For this review, take the finished solid that the model builds, in its own axes (mm). A direction names the side the tool comes from. Round coordinates to 2 decimals unless told otherwise and drop trailing zeros. Order: outer loops, then holes, each group sorted by start corner. A loop starts at its lowest first (then second) coordinate and runs counter-clockwise, first axis right, second up. Notation, with made-up numbers: M 47.25,27 L 75.25,27 A14 cw 75.25,43 Z; hole C 34,71 d3. An arc over 180 degrees is marked long. Put each result on its own line as item: value.
from build123d import *

# Parameters (mm, degrees)
ESQUISSE2_R               = 3.5
ESQUISSE2_R_2             = 1.25
ESQUISSE2_R_3             = 1.5
ESQUISSE2_W               = 8
ESQUISSE2_H               = 3
ESQUISSE2_W_2             = 5.5
T_LE_DE_BASE_PLI_E1_DEPTH = 3


# Sheet-metal steps are written as plain solids
with BuildPart() as part:
    # Esquisse2 → Tôle de base pliée1 (new body)
    with BuildSketch(Plane.XY):
        with BuildLine():
            Line((-80.674813436, 13.65), (-5.9, 13.65))
            ThreePointArc((-5.9, 13.65), (0, 7.75), (-5.9, 1.85))
            Line((-5.9, 1.85), (-80.674813436, 1.85))
            ThreePointArc((-80.674813436, 1.85), (-85.688411127, 8.665e-06), (-90.707519116, 1.834997692))
            ThreePointArc((-90.707519116, 1.834997692), (-94.311259808, 3.720569786), (-98.375041782, 3.887917208))
            ThreePointArc((-98.375041782, 3.887917208), (-102.999999988, 7.750307003), (-98.374437627, 11.611973247))
            ThreePointArc((-98.374437627, 11.611973247), (-94.311297529, 11.778940178), (-90.708236779, 13.664394674))
            ThreePointArc((-90.708236779, 13.664394674), (-85.688881301, 15.499992024), (-80.674813436, 13.65))
        make_face()
        with Locations((-85.7, 7.75)):
            Circle(ESQUISSE2_R, mode=Mode.SUBTRACT)
        with Locations((-5.75, 7.75)):
            Circle(ESQUISSE2_R_2, mode=Mode.SUBTRACT)
        with Locations((-49.7, 7.75)):
            Circle(ESQUISSE2_R_3, mode=Mode.SUBTRACT)
        with Locations((-20, 7.75)):
            Rectangle(ESQUISSE2_W, ESQUISSE2_H, mode=Mode.SUBTRACT)
        with Locations((-60.25, 7.75)):
            Rectangle(ESQUISSE2_W_2, ESQUISSE2_H, mode=Mode.SUBTRACT)
        with BuildLine():
            Line((-75.5, 8.75), (-71, 8.75))
            ThreePointArc((-71, 8.75), (-70, 7.75), (-71, 6.75))
            Line((-71, 6.75), (-75.5, 6.75))
            ThreePointArc((-75.5, 6.75), (-76.5, 7.75), (-75.5, 8.75))
        make_face(mode=Mode.SUBTRACT)
        with BuildLine():
            Line((-99.5, 8.75), (-95.9, 8.75))
            ThreePointArc((-95.9, 8.75), (-94.9, 7.75), (-95.9, 6.75))
            Line((-95.9, 6.75), (-99.5, 6.75))
            ThreePointArc((-99.5, 6.75), (-100.5, 7.75), (-99.5, 8.75))
        make_face(mode=Mode.SUBTRACT)
    extrude(amount=-T_LE_DE_BASE_PLI_E1_DEPTH)


solid = part.part
(1) Add section D-D on x = -79. Give the boundary of the cut face in (y, z).
A:
outline: M 1.85,-3 L 13.65,-3 L 13.65,0 L 1.85,0 Z
(2) Add section C-C on z = -2.1. Give the boundary of the cut face in (x, y) (3 decimals).
A:
outline: M -98.375,3.888 A9.3 cw -90.708,1.835 A7.75 ccw -80.675,1.85 L -5.9,1.85 A5.9 ccw -5.9,13.65 L -80.675,13.65 A7.75 ccw -90.708,13.664 A9.296 cw -98.374,11.612 A3.925 ccw long Z; hole M -99.5,6.75 L -95.9,6.75 A1 ccw -95.9,8.75 L -99.5,8.75 A1 ccw Z; hole C -85.7,7.75 d7; hole M -75.5,6.75 L -71,6.75 A1 ccw -71,8.75 L -75.5,8.75 A1 ccw Z; hole M -63,6.25 L -57.5,6.25 L -57.5,9.25 L -63,9.25 Z; hole C -49.7,7.75 d3; hole M -24,6.25 L -16,6.25 L -16,9.25 L -24,9.25 Z; hole C -5.75,7.75 d2.5
(3) Insertion check: pin 1 Ø1.5 at (x, y) = (-87, 10) entering from +Z; pin 2 Ø0.9 at (x, z) = (-22, -2) entering from -Y; pin 3 Ø1.5 at (x, z) = (-59.5, -2) entering from +Y; pin 4 Ø1.5 at (x, z) = (-98.5, -1) entering from -Y (3 decimals). Each pin has a flat end and moves straight along its axis. Give the tip position at first contact, or say it passes through.
A:
pin 1: passes through
pin 2: stops at y = 1.85
pin 3: stops at y = 13.65
pin 4: stops at y = 3.825
(4) Add section A-A on x = -49.7. Give the boundary of the cut face in (y, z), then the cut area to 3 significant figures.
A:
outline: M 1.85,-3 L 6.25,-3 L 6.25,0 L 1.85,0 Z; M 9.25,-3 L 13.65,-3 L 13.65,0 L 9.25,0 Z
area: 26.4 mm2
(5) To check wall thickness, follow L1, parallel to Y at x = -5.75, z = -1.2; L2, parallel to Y at x = -58.5, z = -1.3; L3, parallel to Y at x = -24.5, z = -0.8. State the ranges of each line that lie inside material, in increasing order.
A:
L1: y = 1.85 to 6.5, 9 to 13.65
L2: y = 1.85 to 6.25, 9.25 to 13.65
L3: y = 1.85 to 13.65
(6) Draft analysis for pull direction Y (two halves, no side actions). For faces 1 (the face through (-48.314, 7.175, -1.479)), 2 (the face through (-103, 7.7, -1.5)), 3 (the face through (-60, 9.25, -1)), 4 (the face through (-51, 10, 0)), state which applies: released by +Y, released by -Y, zero draft, split by the parting line, or undercut.
A:
face 1: undercut
face 2: split by the parting line
face 3: undercut
face 4: zero draft
(7) For faces 5 (the face through (-51, 10, -3)), 6 (the face through (-20, 6.25, -1)), 7 (the face through (-44, 13.65, -1)), list the 3-axis set-ups (+Z, -Z, +X, -X, +Y, -Y) from which the entire face can be reached by the end or side of a thin tool; tool diameter is ignored.
A:
face 5: -Z, +X, -X, +Y, -Y
face 6: +Z, -Z
face 7: +Z, -Z, +X, +Y
(8) Add section B-B on y = 10.25. Give the boundary of the cut face in (x, z).
A:
outline: M -102.1,-3 L -88.15,-3 L -88.15,0 L -102.1,0 Z; M -83.25,-3 L -0.56,-3 L -0.56,0 L -83.25,0 Z
